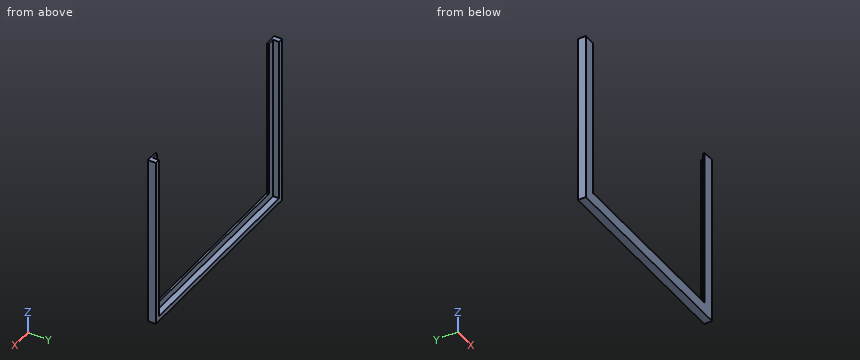
```python
from build123d import *

# Parameters (mm, degrees)
SKETCH1_W               = 206.5
SKETCH1_H               = 350
SKETCH1_W_2             = 182.5
SKETCH1_H_2             = 326
BOSS_EXTRUDE1_DEPTH     = 2
SKETCH2_W               = 206.5
SKETCH2_H               = 350
SKETCH2_W_2             = 196.5
SKETCH2_H_2             = 340
BOSS_EXTRUDE2_DEPTH     = 6
CUT_EXTRUDE3_DEPTH      = 204.345918326
CUT_EXTRUDE3_DEPTH_BACK = 204.345918326
SKETCH3_W               = 400
SKETCH3_H               = 400


with BuildPart() as part:
    # Sketch1 → Boss-Extrude1 (new body)
    with BuildSketch(Plane(origin=(0, 0, 0), x_dir=(1, 0, 0), z_dir=(0, 1, 0))):
        Rectangle(SKETCH1_W, SKETCH1_H)
        Rectangle(SKETCH1_W_2, SKETCH1_H_2, mode=Mode.SUBTRACT)
    extrude(amount=BOSS_EXTRUDE1_DEPTH)

    # Sketch2 → Boss-Extrude2 (add)
    with BuildSketch(Plane(origin=(0, 2, 0), x_dir=(1, 0, 0), z_dir=(0, 1, 0))):
        Rectangle(SKETCH2_W, SKETCH2_H)
        Rectangle(SKETCH2_W_2, SKETCH2_H_2, mode=Mode.SUBTRACT)
    extrude(amount=BOSS_EXTRUDE2_DEPTH)

    # Sketch3 → Cut-Extrude3 (cut, two sides: drawn at the far end of the back side and taken through both)
    with BuildSketch(Plane(origin=(0, 0, 0), x_dir=(1, 0, 0), z_dir=(0, 1, 0)).offset(-CUT_EXTRUDE3_DEPTH_BACK)):
        with Locations((0, -200)):
            Rectangle(SKETCH3_W, SKETCH3_H)
    extrude(amount=CUT_EXTRUDE3_DEPTH + CUT_EXTRUDE3_DEPTH_BACK, mode=Mode.SUBTRACT)


solid = part.part
```
Part model, mm, in its own coordinate system. Round coordinates to 2 decimals unless told otherwise and drop trailing zeros. Order: outer loops, then holes, each group sorted by start corner. A loop starts at its lowest first (then second) coordinate and runs counter-clockwise, first axis right, second up. Notation, with made-up numbers: M -37.75,10 L 19.25,10 A16 cw 19.25,22 Z; hole C 29.5,-13 d10. An arc over 180 degrees is marked long. Put each result on its own line as item: value. Start each with the question number.
1. Drop a flat-ended pin along its axis: pin 1 (0.6 mm diameter, centred on x = 29, y = 1.5, fed in from +Z). Give the stop position or say it passes through.
2. Slice it at A-A on z = -62.5. List the corners of the cut face in (x, y), then the cut area to 3 significant figures.
3. Slice it at B-B on x = -65. List the corners of the cut face in (y, z), then the cut area to 3 significant figures.
4. Drill centre lines: probe 1 along X at (y, z) = (7.25, -77.5); probe 2 along X at (y, z) = (1.5, -79); probe 3 along Z at (x, y) = (-51, 6.5). Where is each one in solid material? Low to high. Write a range as [from, to].
5. Slice it at C-C on y = 3.5. List the corners of the cut face in (x, z).
Findings:
1. pin 1: z = -163
2. outline: M -103.25,0 L -91.25,0 L -91.25,2 L -98.25,2 L -98.25,8 L -103.25,8 Z; M 91.25,0 L 103.25,0 L 103.25,8 L 98.25,8 L 98.25,2 L 91.25,2 Z
2. area: 108 mm2
3. outline: M 0,-175 L 8,-175 L 8,-170 L 2,-170 L 2,-163 L 0,-163 Z
3. area: 54.0 mm2
4. probe 1: [-103.25, -98.25], [98.25, 103.25]
4. probe 2: [-103.25, -91.25], [91.25, 103.25]
4. probe 3: [-175, -170]
5. outline: M -103.25,-175 L 103.25,-175 L 103.25,0 L 98.25,0 L 98.25,-170 L -98.25,-170 L -98.25,0 L -103.25,0 Z
